Autodesk Inventor part; units mm, degrees
ref_plane "YZ Plane" through (0, 0, 0) normal (1, 0, 0) x (0, 1, 0)
ref_plane "XZ Plane" through (0, 0, 0) normal (0, 1, 0) x (-1, 0, 0)
ref_plane "XY Plane" through (0, 0, 0) normal (0, 0, 1) x (1, 0, 0)
sketch "Sketch3" plane through (0, 0, 0) normal (0, 0, 1) x (1, 0, 0)
  line L0 (-1.5, 30.2485) -> (1.5, 30.2485)
  line L1 (1.5, 30.2485) -> (1.5, -30.2485)
  line L2 (1.5, -30.2485) -> (-1.5, -30.2485)
  line L3 (-1.5, -30.2485) -> (-1.5, 30.2485)
  line L4 (1.5, -28.2515) -> (26, -38.4996)
  line L5 (26, -38.4996) -> (26, -41.7515)
  line L6 (26, -41.7515) -> (-1.5, -30.2485)
  point P0 (0, 0)
  point P1 (0, 30.2485)
  point P2 (1.5, 0)
  dimension "d20" = 3
  dimension "d26" = 24.5
  dimension "d39" = 3
  dimension "d41" = 58.5
  dimension "d43" = 72
extrude "Extrusion3" add sketch "Sketch3" along normal blind 170
sketch "Sketch4" plane through (1.5, -28.2515, 0) normal (1, 0, 0) x (0, 0, -1)
  circle A0 centre (-85, 48.031) radius 1.345
  circle A1 centre (-85, 31.369) radius 1.345
  circle A2 centre (-76.669, 39.7) radius 1.345
  circle A3 centre (-93.331, 39.7) radius 1.345
  line L0 (0, 58.5) -> (0, 0)
  line L1 (0, 58.5) -> (-170, 58.5)
  line L2 (-170, 0) -> (-170, 58.5)
  line L3 (0, 0) -> (-170, 0)
  point P0 (-85, 58.5)
  dimension "d28" = 2.69
  dimension "d30" = 8.331
  dimension "d31" = 8.331
  dimension "d32" = 8.331
  dimension "d33" = 8.331
  dimension "d34" = 16.662
  dimension "d35" = 16.662
  dimension "d36" = 10.469
extrude "Extrusion4" cut sketch "Sketch4" against normal through all contours A0 | A1 | A2 | A3
fillet "Fillet1" radius 2 1 edges at (1.5, -28.2515, 85)
equation "\"d31\" = d30"
equation "\"d32\" = d30"
equation "\"d33\" = d30"
equation "\"d35\" = d34"
properties part number "CowCatcherRearShort"
Here's how the part is built. I have some questions about the finished solid (model axes, mm). A direction names the side the tool comes from. Coordinates: 2 decimals unless noted, no trailing zeros. Order: outer loops, then holes, each group sorted by start corner. A loop starts at its lowest first (then second) coordinate and runs counter-clockwise, first axis right, second up. Notation, with made-up numbers: (-13, 46.5) -> (37, 46.5) arc R29 ccw to (37, 78.5) -> close; hole circle Ø11 at (52, 18.5). An arc over 180 degrees is marked (long way). Return JSON: item names as keys, results as strings.
1) If we section it at C-C on x = 15.75: List the corners of the cut face in (y, z) for me, plus the area to 3 significant figures.
Conclusion:
{"outline": "(-37.46, 0) -> (-34.21, 0) -> (-34.21, 170) -> (-37.46, 170) -> close", "area": "553 mm²"}
2) On a 3-axis mill with a long thin cutter (end or side, diameter ignored), from which of +Z, -Z, +X, -X, +Y, -Y can I reach the whole of each face in a straight line? I mean faces 1 (the flat face through (26, -40, 84)), 2 (the flat face through (1.5, 2, 84)). Say none if no direction works.
Conclusion:
{"face 1": "+Z, -Z, +X, +Y, -Y", "face 2": "+Z, -Z, +X, +Y"}
3) If we section it at A-A on z = 13: List the corners of the cut face in (x, y) for me, plus the area to 3 significant figures.
Conclusion:
{"outline": "(-1.5, -30.25) -> (26, -41.75) -> (26, -38.5) -> (2.73, -28.77) arc R2 cw to (1.5, -26.92) -> (1.5, 30.25) -> (-1.5, 30.25) -> close", "area": "263 mm²"}
4) If we section it at B-B on y = 8: List the corners of the cut face in (x, z) for me.
Conclusion:
{"outline": "(-1.5, 0) -> (1.5, 0) -> (1.5, 170) -> (-1.5, 170) -> close"}
5) I'm going to push flat-ended pins straight in: P1, Ø12, axis at x = 7.5, z = 44, coming from the -Y side; P2, Ø1.6, axis at y = 11.45, z = 76.67, coming from the +X side; P3, Ø3, axis at x = 14.5, z = 38, coming from the -Y side; P4, Ø1, axis at x = 16, z = 71, coming from the +Y side. Where does each tip first touch, or does it pass through?
Conclusion:
{"P1": "stops at y = -36.52", "P2": "passes through", "P3": "stops at y = -37.57", "P4": "stops at y = -34.11"}
6) If I drill on probe 1 along Y at (x, z) = (0, 85); probe 2 along X at (y, z) = (-2, 47); probe 3 along Y at (x, z) = (6, 95), over which ranges is the centre line in solid material (lowest first)?
Conclusion:
{"probe 1": "y = -30.88 to 1.77, 4.46 to 18.43, 21.12 to 30.25", "probe 2": "x = -1.5 to 1.5", "probe 3": "y = -33.39 to -30.13"}
